from build123d import *

# Parameters (mm, degrees)
F1_DEPTH = 0.8


with BuildPart() as f1:
    # F0 (on Right) → F1 (new body)
    with BuildSketch(Plane.YZ):
        with BuildLine():
            ThreePointArc((-4.788236, 5), (-8.32377, 3.535534), (-9.788236, 0))
            Line((-9.788236, 0), (-9.788236, -25))
            Line((-9.788236, -25), (10.211764, -25))
            Line((10.211764, -25), (10.211764, 5))
            Line((10.211764, 5), (-4.788236, 5))
        make_face()
    extrude(amount=F1_DEPTH)


solid = f1.part
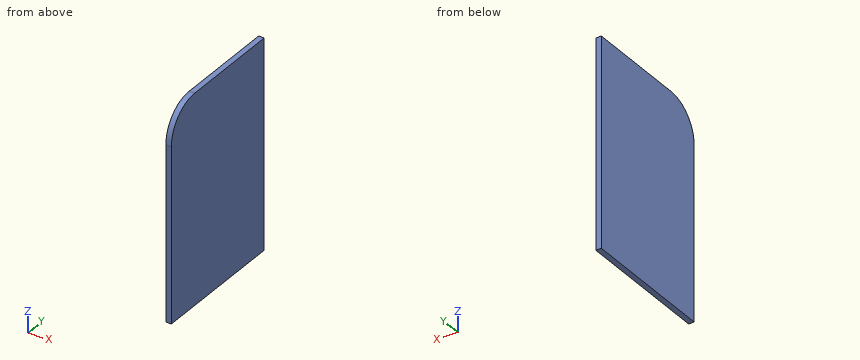
Check sheet for the modelled part. Datum: model origin and axes. Units: mm. Give positions to 0.01 mm unless a question says otherwise; leave off trailing zeros. Loops run counter-clockwise (first coordinate to the right, second up) from the corner with the lowest first, then second, coordinate; pieces in that order, holes last. Notation, with made-up numbers: M 30.5,2 L 62.5,2 A24 ccw 62.5,28 Z; hole C -19.5,63 d6. An arc over 180 degrees is marked long. Answer as a JSON object with one key per item and string values. Group by question number.
Q1. Material ranges on line 1 along Y through (x, z) = (0.25, 0.5); line 2 along Z through (x, y) = (0.1, -5.75); line 3 along Z through (x, y) = (0.15, -5.25), recorded low to high. Write a range as [from, to].
Q2. Cross-section at A-A on z = 2. Record the cut outline in (x, y).
Q3. Cross-section at B-B on y = -7.5. Record the cut outline in (x, z).
Evaluation:
{
 "1": {"line 1": "y = [-9.76, 10.21]", "line 2": "z = [-25, 4.91]", "line 3": "z = [-25, 4.98]"},
 "2": {"outline": "M 0,-9.37 L 0.8,-9.37 L 0.8,10.21 L 0,10.21 Z"},
 "3": {"outline": "M 0,-25 L 0.8,-25 L 0.8,4.2 L 0,4.2 Z"}
}
